Solid Edge part; units mm, degrees
sketch "Sketch1" plane through (0, 0, 0) normal (0, 0, 1) x (1, 0, 0)
  line L0 (-22.75, -10) -> (22.75, -10)
  line L1 (22.75, -10) -> (22.75, 10)
  line L2 (22.75, 10) -> (-22.75, 10)
  line L3 (-22.75, 10) -> (-22.75, -10)
  dimension "D1" = 22.75
  dimension "D2" = 22.75
extrude "Protrusion1" add sketch "Sketch1" along normal blind 1.7
sketch "Sketch2" plane through (0, 0, 1.7) normal (0, 0, 1) x (1, 0, 0)
  circle A0 centre (-12.9, 0) radius 8
  circle A1 centre (12.9, 0) radius 8
extrude "ProtrusiónExtruida_2" add sketch "Sketch2" along normal blind 12
sketch "Sketch3" plane through (0, 0, 1.7) normal (0, 0, 1) x (1, 0, 0)
  line L0 (-2.8632, 9) -> (2.8632, 9)
  arc A0 (2.8632, 9) -> (2.8632, 5.5) centre (2.8632, 7.25) cw
  line L1 (2.8632, 5.5) -> (-2.8632, 5.5)
  arc A1 (-2.8632, 5.5) -> (-2.8632, 9) centre (-2.8632, 7.25) cw
extrude "ProtrusiónExtruida_3" add sketch "Sketch3" along normal blind 3.2
sketch "Sketch4" plane through (0, 0, 0) normal (0, 0, -1) x (-1, 0, 0)
  line L0 (-5.2, -9.5) -> (5.2, -9.5)
  line L1 (5.2, -9.5) -> (5.2, -6.9)
  line L2 (5.2, -6.9) -> (-5.2, -6.9)
  line L3 (-5.2, -6.9) -> (-5.2, -9.5)
  dimension "D1" = 5.2
  dimension "D2" = 5.2
extrude "ProtrusiónExtruida_6" add sketch "Sketch4" along normal blind 2.6
sketch "Sketch5" plane through (0, -8.2, -2.6) normal (0, 0, -1) x (-1, 0, 0)
  line L0 (-4.2, -0.65) -> (-3, -0.65)
  line L1 (-3, -0.65) -> (-3, 0.65)
  line L2 (-3, 0.65) -> (-4.2, 0.65)
  line L3 (-4.2, 0.65) -> (-4.2, -0.65)
  line L4 (-1.8, -0.65) -> (-0.6, -0.65)
  line L5 (-0.6, -0.65) -> (-0.6, 0.65)
  line L6 (-0.6, 0.65) -> (-1.8, 0.65)
  line L7 (-1.8, 0.65) -> (-1.8, -0.65)
  line L8 (0.6, -0.6308) -> (1.8, -0.6308)
  line L9 (1.8, -0.6308) -> (1.8, 0.65)
  line L10 (1.8, 0.65) -> (0.6, 0.65)
  line L11 (0.6, 0.65) -> (0.6, -0.6308)
  line L12 (3, -0.6308) -> (4.2, -0.6308)
  line L13 (4.2, -0.6308) -> (4.2, 0.65)
  line L14 (4.2, 0.65) -> (3, 0.65)
  line L15 (3, 0.65) -> (3, -0.6308)
  dimension "D1" = 3
  dimension "D2" = 4.2
extrude "ProtrusiónExtruida_8" add sketch "Sketch5" along normal blind 1.9
sketch "Sketch6" plane through (-3.6, -8.8308, -3.55) normal (0, -1, 0) x (-1, 0, 0)
  line L0 (-7.8, -0.0931) -> (-6.6, -0.0931)
  line L1 (-6.6, -0.0931) -> (-6.6, 0.95)
  line L2 (-6.6, 0.95) -> (-7.8, 0.95)
  line L3 (-7.8, 0.95) -> (-7.8, -0.0931)
  line L4 (-5.4, -0.0931) -> (-4.2, -0.0931)
  line L5 (-4.2, -0.0931) -> (-4.2, 0.95)
  line L6 (-4.2, 0.95) -> (-5.4, 0.95)
  line L7 (-5.4, 0.95) -> (-5.4, -0.0931)
  line L8 (-3, -0.0931) -> (-1.8, -0.0931)
  line L9 (-1.8, -0.0931) -> (-1.8, 0.95)
  line L10 (-1.8, 0.95) -> (-3, 0.95)
  line L11 (-3, 0.95) -> (-3, -0.0931)
  line L12 (-0.6, -0.0931) -> (0.6, -0.0931)
  line L13 (0.6, -0.0931) -> (0.6, 0.95)
  line L14 (0.6, 0.95) -> (-0.6, 0.95)
  line L15 (-0.6, 0.95) -> (-0.6, -0.0931)
extrude "ProtrusiónExtruida_9" add sketch "Sketch6" along normal blind 7.2
fillet "Redondeo_1" radius 0.5 8 edges at (3.6, -7.55, -4.5) (1.2, -7.55, -4.5) (-1.2, -7.55, -4.5) (-3.6, -7.55, -4.5) (3.6, -8.85, -3.4569) (1.2, -8.85, -3.4569) (-1.2, -8.8308, -3.4569) (-3.6, -8.8308, -3.4569)
hole "Agujero_1" at (-21.2, 8.6, 1.7) direction (0, 0, -1) diameter 1.6 end up to next
hole "Hole1" at (-21.2, -8.45, 1.7) direction (0, 0, -1) diameter 1.6 end up to next
hole "Hole2" at (21.2, 8.6, 1.7) direction (0, 0, -1) diameter 1.6 end up to next
hole "Hole3" at (21.2, -8.45, 1.7) direction (0, 0, -1) diameter 1.6 end up to next
Verification items for the finished model (mm, model axes). A direction names the side the tool comes from. Coordinates: 2 decimals unless noted, no trailing zeros. Order: outer loops, then holes, each group sorted by start corner. A loop starts at its lowest first (then second) coordinate and runs counter-clockwise, first axis right, second up. Notation, with made-up numbers: (33.5, -7) -> (48.5, -7) arc R15 ccw to (48.5, 22) -> close; hole circle Ø6 at (-33, 68). An arc over 180 degrees is marked (long way). Use CSV: the item, a comma, the result in double quotes. Start each with the question number.
Q1. Section check D-D, the plane z = 9.25. Record the cut outline in (x, y).
Q2. Draft check along X on faces 4 (the flat face through (0, 7, 4.9)), 5 (the flat face through (-22.75, 0, 1)), 6 (the flat face through (4, -12, -4.5)). Enter one of: +X half, -X half, draft (parallel to the pull), parting line (faces both ways), or undercut.
Q3. Section check B-B, the plane x = -12.9. Record the cut outline in (y, z).
Q4. Section check A-A, the plane z = 3. Record the cut outline in (x, y).
Q5. Thickness scan on line 1 along Y through (x, z) = (-21.2, 0.8); line 2 along X through (y, z) = (8.6, 0.75); line 3 along Z through (x, y) = (14.5, -4.25). Record the ranges inside material, lowest first.
Q6. Section check C-C, the plane y = -4.25. Record the cut outline in (x, z).
Q7. Depth check by flat-ended pin: P1, Ø4, axis at x = -0.5, y = 7.5, coming from the +Z side; P2, Ø0.6, axis at y = -13, z = -4, coming from the +X side; P3, Ø0.6, axis at x = 4, z = -3, coming from the +Y side; P4, Ø2, axis at y = 5.5, z = -2.5, coming from the -X side. Enter the tip coordinate at first touch or a pass-through.
Q8. Tool access check on faces 1 (the flat face through (0, -9.5, -1)), 2 (the flat face through (5.2, -8, -1)), 3 (the flat face through (0, -6.9, -1)). Record the directions out of +Z, -Z, +X, -X, +Y, -Y that give a thin tool (end or side, any length) a straight path to the whole face; none if there is none.
Returned:
1,outline,"circle Ø16 at (-12.9, 0); circle Ø16 at (12.9, 0)"
2,face 4,"undercut"
2,face 5,"-X half"
2,face 6,"draft"
3,outline,"(-10, 0) -> (10, 0) -> (10, 1.7) -> (8, 1.7) -> (8, 13.7) -> (-8, 13.7) -> (-8, 1.7) -> (-10, 1.7) -> close"
4,outline,"circle Ø16 at (-12.9, 0); (-2.86, 5.5) -> (2.86, 5.5) arc R1.75 ccw to (2.86, 9) -> (-2.86, 9) arc R1.75 ccw to start; circle Ø16 at (12.9, 0)"
5,line 1,"y = -10 to -9.25, -7.65 to 7.8, 9.4 to 10"
5,line 2,"x = -22.75 to -22, -20.4 to 20.4, 22 to 22.75"
5,line 3,"z = 0 to 13.7"
6,outline,"(-22.75, 0) -> (22.75, 0) -> (22.75, 1.7) -> (19.68, 1.7) -> (19.68, 13.7) -> (6.12, 13.7) -> (6.12, 1.7) -> (-6.12, 1.7) -> (-6.12, 13.7) -> (-19.68, 13.7) -> (-19.68, 1.7) -> (-22.75, 1.7) -> close"
7,P1,"stops at z = 4.9"
7,P2,"stops at x = 4.2"
7,P3,"stops at y = -7.55"
7,P4,"passes through"
8,face 1,"+X, -X, -Y"
8,face 2,"-Z, +X, +Y, -Y"
8,face 3,"-Z, +X, -X, +Y"
